Geometry: final body of the model. Coordinates: model frame, mm. A direction names the side the tool comes from. Round coordinates to 2 decimals unless told otherwise and drop trailing zeros. Write each loop counter-clockwise with the first axis right and the second up, starting at its lowest first coordinate (ties: lowest second). Pieces come first, ordered by that corner, then holes.
from build123d import *

# Parameters (mm, degrees)
F1_DEPTH = 38.1
F2_R     = 1.524
F3_R     = 1.5875
F3_R_2   = 2.54
F4_DEPTH = 2.54
F6_DEPTH = 2.54
F7_R     = 6.35
F8_W     = 157.243733
F8_H     = 94.123651
F9_DEPTH = 19.05
F10_R    = 1.524


with BuildPart() as f1:
    # F0 (on Right) → F1 (new body)
    with BuildSketch(Plane.YZ):
        with BuildLine():
            Line((-54.864, 1.016), (-52.324, 1.016))
            Line((-52.324, 1.016), (-52.324, 41.402))
            ThreePointArc((-52.324, 41.402), (-51.877631, 42.479631), (-50.8, 42.926))
            Line((-50.8, 42.926), (-0.254, 42.926))
            Line((-0.254, 42.926), (-0.254, 45.466))
            Line((-0.254, 45.466), (-50.8, 45.466))
            ThreePointArc((-50.8, 45.466), (-53.673682, 44.275682), (-54.864, 41.402))
            Line((-54.864, 41.402), (-54.864, 1.016))
        make_face()
    extrude(amount=F1_DEPTH)

    # F2
    f2_edges = [f1.edges().sort_by_distance(p)[0] for p in [
        (0, -0.254, 44.196),
        (38.1, -0.254, 44.196),
    ]]
    fillet(f2_edges, radius=F2_R)

    # F3 (on face) → F4 (cut, through all)
    with BuildSketch(Plane(origin=(0, 0, 42.926), x_dir=(1, 0, 0), z_dir=(0, 0, -1))):
        with Locations((6.1595, 43.7515)):
            Circle(F3_R)
        with Locations((19.05, 39.624)):
            Circle(F3_R_2)
        with Locations((31.9405, 43.7515)):
            Circle(F3_R)
        with Locations((19.05, 7.874)):
            Circle(F3_R_2)
    extrude(amount=-F4_DEPTH, mode=Mode.SUBTRACT)

    # F5 (on face) → F6 (cut, through all)
    with BuildSketch(Plane.XZ.offset(54.864)):
        with BuildLine():
            ThreePointArc((13.97, 7.874), (14.044395, 7.694395), (14.224, 7.62))
            Line((14.224, 7.62), (23.876, 7.62))
            ThreePointArc((23.876, 7.62), (24.055605, 7.694395), (24.13, 7.874))
            Line((24.13, 7.874), (24.13, 16.891))
            ThreePointArc((24.13, 16.891), (24.055605, 17.070605), (23.876, 17.145))
            Line((23.876, 17.145), (14.224, 17.145))
            ThreePointArc((14.224, 17.145), (14.044395, 17.070605), (13.97, 16.891))
            Line((13.97, 16.891), (13.97, 7.874))
        make_face()
    extrude(amount=-F6_DEPTH, mode=Mode.SUBTRACT)

    # F7
    f7_edges = [f1.edges().sort_by_distance(p)[0] for p in [
        (38.1, -53.594, 1.016),
        (0, -53.594, 1.016),
    ]]
    fillet(f7_edges, radius=F7_R)

    # F8 (on face) → F9 (cut)
    with BuildSketch(Plane(origin=(0, -0.254, 0), x_dir=(-1, 0, 0), z_dir=(0, 1, 0))):
        with Locations((-60.055602, 67.589141)):
            Rectangle(F8_W, F8_H)
    extrude(amount=-F9_DEPTH, mode=Mode.SUBTRACT)

    # F10
    f10_edges = [f1.edges().sort_by_distance(p)[0] for p in [
        (38.1, -19.304, 44.196),
        (0, -19.304, 44.196),
    ]]
    fillet(f10_edges, radius=F10_R)


solid = f1.part
1) Draft query along Y for faces 1 (the cylindrical face through (18.719, -42.142, 44.178)), 2 (the flat face through (19, -54.864, 21)), 3 (the cylindrical face through (31.6, -42.2, 44.2)), 4 (the flat face through (19, -19.304, 44)). Return one class per face: pulls with the +Y half, pulls with the -Y half, needs draft (parallel to the pull), parting line crosses it, or undercut.
2) Section C-C on y = -22.5. Output: boundary loops of the cut face in (x, z).
3) Line query: probe 1 along Y at (x, z) = (35.5, 29); probe 2 along Z at (x, y) = (20.5, -31); probe 3 along Y at (x, z) = (19, 44). Output: solid intervals per line, ascending.
4) Section D-D on z = 30. Output: boundary loops of the cut face in (x, y), plus the area to 3 significant figures.
5) Reachability of faces 5 (the flat face through (19, -35, 42.926)), 6 (the flat face through (24.13, -54, 12)), 7 (the cylindrical face through (0.4, -19.8, 44.2)) from +Z, -Z, +X, -X, +Y, -Y: full face, straight path, thin tool, end or side. Return the list, or none.
6) Section A-A on x = 19.05. Output: boundary loops of the cut face in (y, z) (3 decimals).
7) Section B-B on x = 27.5. Output: boundary loops of the cut face in (y, z), plus the area to 3 significant figures.
8) First-contact query: P1, Ø1.5, axis at x = 28, z = 18.5, coming from the +Y side; P2, Ø0.8, axis at x = 21, y = -53.5, coming from the +Z side; P3, Ø12, axis at x = 21, y = -41.5, coming from the -Z side; P4, Ø3, axis at y = -50, z = 36, coming from the +X side. Flat tips, straight axial feed; report the tip coordinate or a pass-through.
Filled in:
1. face 1: undercut
1. face 2: pulls with the -Y half
1. face 3: undercut
1. face 4: pulls with the +Y half
2. outline: (0, 42.93) - (38.1, 42.93) - (38.1, 45.47) - (0, 45.47) - close
3. probe 1: y = -54.86 to -52.32
3. probe 2: z = 42.93 to 45.47
3. probe 3: y = -53.93 to -42.16, -37.08 to -19.3
4. outline: (0, -54.86) - (38.1, -54.86) - (38.1, -52.32) - (0, -52.32) - close
4. area: 96.8 mm2
5. face 5: -Z, +X, -X, +Y
5. face 6: +Y, -Y
5. face 7: +Z, -Z, -X, +Y
6. outline: (-54.864, 1.016) - (-52.324, 1.016) - (-52.324, 7.62) - (-54.864, 7.62) - close; (-54.864, 17.145) - (-52.324, 17.145) - (-52.324, 41.402) arc R1.524 cw to (-50.8, 42.926) - (-42.164, 42.926) - (-42.164, 45.466) - (-50.8, 45.466) arc R4.064 ccw to (-54.864, 41.402) - close; (-37.084, 42.926) - (-19.304, 42.926) - (-19.304, 45.466) - (-37.084, 45.466) - close
7. outline: (-54.86, 1.02) - (-52.32, 1.02) - (-52.32, 41.4) arc R1.52 cw to (-50.8, 42.93) - (-19.3, 42.93) - (-19.3, 45.47) - (-50.8, 45.47) arc R4.06 ccw to (-54.86, 41.4) - close
7. area: 194 mm2
8. P1: stops at y = -52.32
8. P2: stops at z = 44.75
8. P3: stops at z = 42.93
8. P4: passes through
